Part model, mm, in its own coordinate system. A direction names the side the tool comes from. Round coordinates to 2 decimals unless told otherwise and drop trailing zeros. Write each loop counter-clockwise with the first axis right and the second up, starting at its lowest first coordinate (ties: lowest second). Pieces come first, ordered by that corner, then holes.
1) Saw through at B-B on z = 5.25. Write the cut outline in (x, y) (3 decimals), and give its area (3 significant figures).
2) Flat gauge pins, fed straight in: pin 1 (2.5 mm diameter, centred on x = -6.35, z = 0, fed in from +Y); pin 2 (5 mm diameter, centred on x = 1, y = -17, fed in from +Z); pin 3 (3 mm diameter, centred on y = 4.5, z = -5.5, fed in from -X). Where does each tip first touch, or does it go through?
3) Which spindle directions (+Z, -Z, +X, -X, +Y, -Y) get a long thin tool onto all of the face, cutting with end or side? Do faces 5 (the flat face through (-8, 25.4, -1)), 6 (the flat face through (0, 0, -5)). Say none if no direction does.
4) Saw through at C-C on x = -0.75. Write the cut outline in (y, z) (3 decimals).
5) Saw through at A-A on x = -6.35. Count the separate pieces of the cut face and the enclosed holes in it, and give its area (3 significant figures).
6) Drill centre lines: L1, parallel to Y at x = -3, z = 3.5 (3 decimals); L2, parallel to X at y = 5.5, z = -5.5; L3, parallel to Z at x = 4.5, y = 13. Where is each one in solid material? Low to high.
7) Saw through at D-D on z = -4.75. Write the cut outline in (x, y) (3 decimals), and give its area (3 significant figures).
8) Pull direction X, two halves, no side cores. Call faces 1 (the flat face through (-12.7, 24, -3)), 2 (the cylindrical face through (-4.836, 23.835, 0.477)), 3 (the flat face through (1, 0, -3.704)), 4 (the cylindrical face through (-4.836, -23.79, 0.477)): +X half, -X half, draft (parallel to the pull), parting line (faces both ways), or undercut.
```python
from build123d import *

# Parameters (mm, degrees)
F0_R     = 1.5875
F1_DEPTH = 25.4
F2_W     = 44.45
F2_H     = 11.1125
F3_DEPTH = 25.4
F4_W     = 12.7
F4_H     = 44.45
F5_DEPTH = 2.646833


with BuildPart() as f1:
    # F0 (on Front) → F1 (new body, symmetric)
    with BuildSketch(Plane.XZ):
        with BuildLine():
            Line((0, -6.35), (6.35, -6.35))
            ThreePointArc((6.35, -6.35), (1.859872, -4.490128), (0, 0))
            ThreePointArc((0, 0), (-6.35, 6.35), (-12.7, 0))
            Line((-12.7, 0), (-12.7, -6.35))
            Line((-12.7, -6.35), (0, -6.35))
        make_face()
        with Locations((-6.35, 0)):
            Circle(F0_R, mode=Mode.SUBTRACT)
    extrude(amount=F1_DEPTH, both=True)

    # F2 (on Right) → F3 (cut, symmetric)
    with BuildSketch(Plane.YZ):
        with Locations((0, 1.852083)):
            Rectangle(F2_W, F2_H)
    extrude(amount=F3_DEPTH, both=True, mode=Mode.SUBTRACT)

    # F4 (on face) → F5 (cut, through all)
    with BuildSketch(Plane.XY.offset(-3.704167)):
        with Locations((-6.35, 0)):
            Rectangle(F4_W, F4_H)
    extrude(amount=-F5_DEPTH, mode=Mode.SUBTRACT)


solid = f1.part
```
Completed:
1. outline: (-9.922, -25.4) - (-2.778, -25.4) - (-2.778, -22.225) - (-9.922, -22.225) - close; (-9.922, 22.225) - (-2.778, 22.225) - (-2.778, 25.4) - (-9.922, 25.4) - close
1. area: 45.4 mm2
2. pin 1: passes through
2. pin 2: stops at z = -3.7
2. pin 3: stops at x = 0
3. face 5: +Z, -Z, +X, -X, +Y
3. face 6: +Z, -Z, -X
4. outline: (-25.4, -6.35) - (-22.225, -6.35) - (-22.225, 2.994) - (-25.4, 2.994) - close; (22.225, -6.35) - (25.4, -6.35) - (25.4, 2.994) - (22.225, 2.994) - close
5. separate pieces: 4
5. enclosed holes: 0
5. area: 60.5 mm2
6. L1: y = -25.4 to -22.225, 22.225 to 25.4
6. L2: x = 0 to 3.18
6. L3: z = -6.35 to -6.07
7. outline: (-12.7, -25.4) - (2.136, -25.4) - (2.136, 25.4) - (-12.7, 25.4) - (-12.7, 22.225) - (0, 22.225) - (0, -22.225) - (-12.7, -22.225) - close
7. area: 189 mm2
8. face 1: -X half
8. face 2: undercut
8. face 3: draft
8. face 4: undercut
